Verification items for this drawing (mm, ordinates from the low corner). Coordinates: 2 decimals unless noted, no trailing zeros. Order: outer loops, then holes, each group sorted by start corner. A loop starts at its lowest first (then second) coordinate and runs counter-clockwise, first axis right, second up. Notation, with made-up numbers: (-37.5, 2) -> (20.5, 2) arc R11 ccw to (20.5, 23) -> close; hole circle Ø2 at (-25, 86). An arc over 180 degrees is marked (long way). Write each question's results on one line, items separated by ' | '. Start each with the question number.
(1) Cross-section at C-C on x = 16.5. Enter the section's corners in (y, z).
(2) Cross-section at D-D on y = 0.5. Enter the section's corners in (x, z) (3 decimals), and give its area (3 significant figures).
(3) Thickness scan on probe 1 along X at (y, z) = (1.2, 52.4) (3 decimals); probe 2 along X at (y, z) = (2.75, 53). Record the ranges inside material, lowest first. Write a range as [from, to].
(4) Cross-section at A-A on x = 52.4. Enter the section's corners in (y, z) (3 decimals), and give its area (3 significant figures).
(5) Go/stop test with a flat-tipped pin: pin 1 (1 mm diameter, centred on x = 63, y = 2.5, fed in from -Z). Record where the tip stops, or that it passes through.
(6) Cross-section at B-B on z = 52.4. Enter the section's corners in (x, y) (3 decimals).
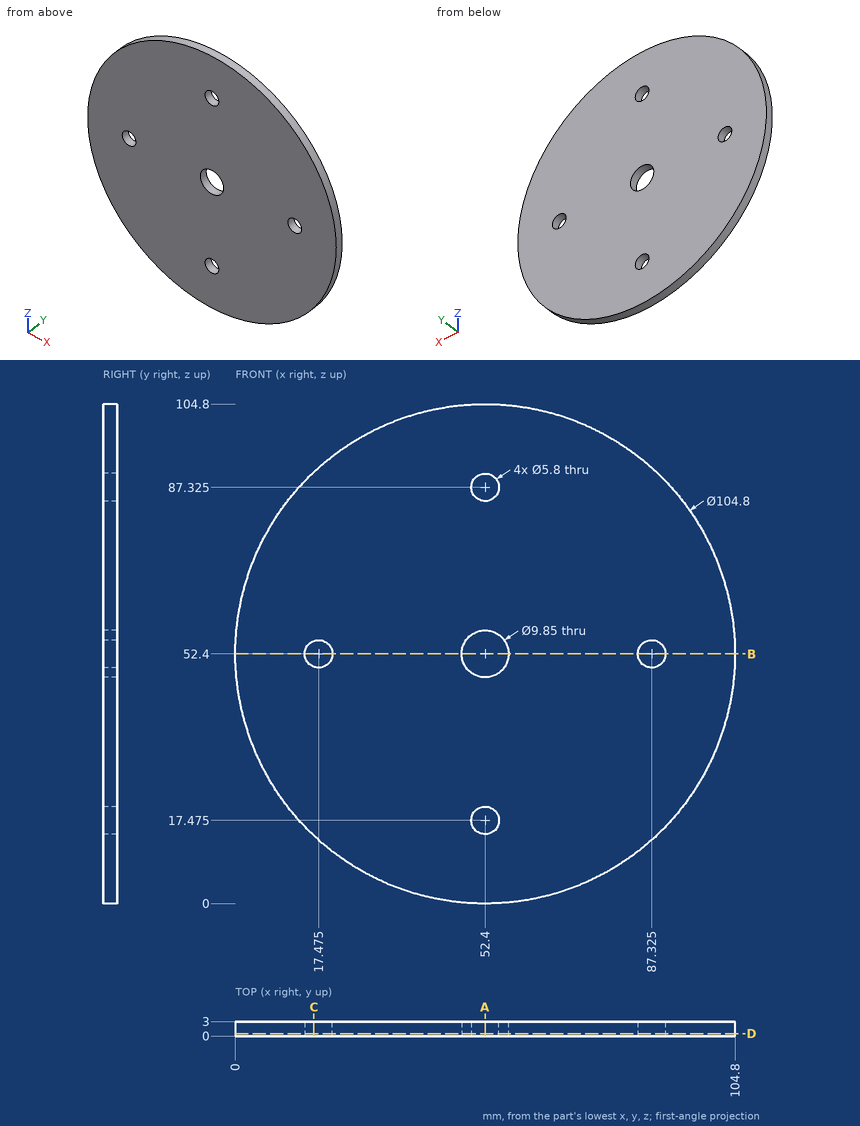
Results are:
1) outline: (0, 14.23) -> (3, 14.23) -> (3, 49.67) -> (0, 49.67) -> close; (0, 55.13) -> (3, 55.13) -> (3, 90.57) -> (0, 90.57) -> close
2) outline: circle Ø104.8 at (52.4, 52.4); hole circle Ø5.8 at (17.475, 52.4); hole circle Ø9.85 at (52.4, 52.4); hole circle Ø5.8 at (52.4, 17.475); hole circle Ø5.8 at (52.4, 87.325); hole circle Ø5.8 at (87.325, 52.4) | area: 8,440 mm2
3) probe 1: x = [0, 14.575], [20.375, 47.475], [57.325, 84.425], [90.225, 104.8] | probe 2: x = [0, 14.64], [20.31, 47.51], [57.29, 84.49], [90.16, 104.8]
4) outline: (0, 0) -> (3, 0) -> (3, 14.575) -> (0, 14.575) -> close; (0, 20.375) -> (3, 20.375) -> (3, 47.475) -> (0, 47.475) -> close; (0, 57.325) -> (3, 57.325) -> (3, 84.425) -> (0, 84.425) -> close; (0, 90.225) -> (3, 90.225) -> (3, 104.8) -> (0, 104.8) -> close | area: 250 mm2
5) pin 1: stops at z = 0.98
6) outline: (0, 0) -> (14.575, 0) -> (14.575, 3) -> (0, 3) -> close; (20.375, 0) -> (47.475, 0) -> (47.475, 3) -> (20.375, 3) -> close; (57.325, 0) -> (84.425, 0) -> (84.425, 3) -> (57.325, 3) -> close; (90.225, 0) -> (104.8, 0) -> (104.8, 3) -> (90.225, 3) -> close
